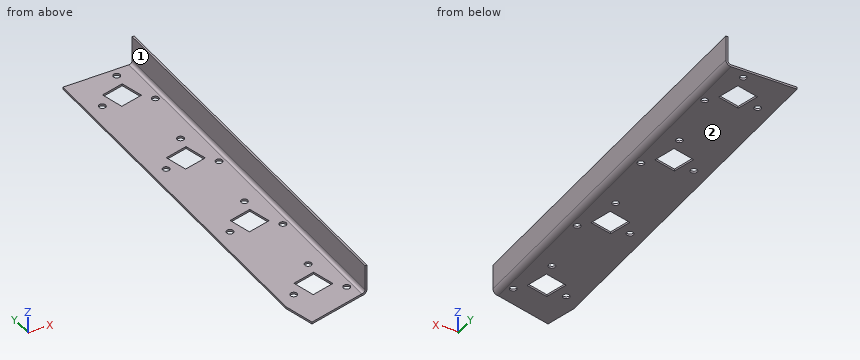
Autodesk Inventor part; units mm, degrees
ref_plane "YZ Plane" through (0, 0, 0) normal (1, 0, 0) x (0, 1, 0)
ref_plane "XZ Plane" through (0, 0, 0) normal (0, 1, 0) x (-1, 0, 0)
ref_plane "XY Plane" through (0, 0, 0) normal (0, 0, 1) x (1, 0, 0)
sketch "Sketch1" plane through (0, 0, 0) normal (0, 0, 1) x (1, 0, 0)
  line L0 (-52.5, 292) -> (52.5, 292)
  line L1 (52.5, 292) -> (52.5, -292)
  line L2 (52.5, -292) -> (-52.5, -292)
  line L3 (-52.5, -292) -> (-52.5, 292)
  line L4 (-52.5, 292) -> (52.5, -292) construction
  point P0 (0, 0)
  point P1 (0, 0)
  dimension "d0" = 105
  dimension "d1" = 584
extrude "Plate1" add sketch "Sketch1" along normal blind 3
sketch "Sketch4" plane through (49.5, 292, 0) normal (1, 0, 0) x (0, 1, 0)
  line L0 (-584, 0) -> (0, 0)
  line L1 (0, 0) -> (0, 45)
  line L2 (0, 45) -> (-584, 45)
  line L3 (-584, 45) -> (-584, 0)
edge flange "Flange1" height 45 angle 90 thickness 3 bend radius 5 thickness toward (1, 0, 0) relief round relief width 3 relief depth 1.5 edges at (52.5, 0, 3) wall of the first edge with corners at (49.5, -292, 0) (49.5, 292, 0) (49.5, 292, 45) (49.5, -292, 45)
bend "Bend1"
corner "Corner1"
sketch "Sketch5" plane through (0, 0, 0) normal (0, 0, -1) x (-1, 0, 0)
  line L0 (-44.5, 292) -> (-44.5, -292)
  line L1 (52.5, -292) -> (-44.5, -292)
  line L2 (52.5, 292) -> (52.5, -292)
  line L3 (-44.5, 292) -> (52.5, 292)
  line L4 (52.5, -292) -> (52.5, -316.1848)
  line L5 (-44.5, -292) -> (52.5, -292)
  line L6 (52.5, -316.1848) -> (-44.5, -292)
  point P0 (0, 0)
  dimension "d25" = 14
extrude "Extrusion2" add sketch "Sketch5" against normal up to surface (3 mm away) contours L1 L4 L6
sketch "Sketch6" plane through (0, 0, 0) normal (0, 0, -1) x (-1, 0, 0)
  line L0 (-44.5, 292) -> (-44.5, -292) construction
  line L1 (-44.5, -292) -> (52.5, -316.1848)
  line L2 (52.5, 292) -> (52.5, -316.1848)
  line L3 (-44.5, 292) -> (52.5, 292) construction
  line L4 (41.1893, -313.3647) -> (52.5, -268)
  line L5 (-44.5, -292) -> (52.5, -316.1848)
  point P0 (0, 0)
  dimension "d45" = 560
extrude "Cut1" cut sketch "Sketch6" against normal blind 3
sketch "Sketch7" plane through (0, 0, 0) normal (0, 0, 1) x (1, 0, 0)
  line L0 (44.5, -292) -> (-41.1893, -313.3647)
  circle A0 centre (36.1472, -268.8326) radius 5.05
  line L1 (36.1472, -268.8326) -> (19.2126, -200.9119) construction
  line L2 (24.6363, -253.6668) -> (16.1691, -219.7064)
  circle A1 centre (19.2126, -200.9119) radius 5.05
  line L3 (-30.5378, -249.3875) -> (36.1472, -268.8326) construction
  line L4 (24.6363, -253.6668) -> (-17.7913, -228.1737) construction
  line L5 (16.1691, -219.7064) -> (-17.7913, -228.1737)
  line L6 (-9.324, -262.1341) -> (24.6363, -253.6668)
  line L7 (16.1691, -219.7064) -> (-9.324, -262.1341) construction
  line L8 (-17.7913, -228.1737) -> (-9.324, -262.1341)
  line L9 (20.4027, -236.6866) -> (-30.5378, -249.3875) construction
  line L10 (19.2126, -200.9119) -> (-30.5378, -249.3875) construction
  circle A2 centre (-30.5378, -249.3875) radius 5.05
  point P0 (0, 0)
  point P1 (3.4225, -240.9203)
  dimension "d32" = 35
  dimension "d33" = 35
  dimension "d34" = 10.1
  dimension "d35" = 70
  dimension "d36" = 60
  dimension "d37" = 25
  dimension "d38" = 10
  dimension "d39" = 42
extrude "Extrusion3" cut sketch "Sketch7" along normal through all
pattern_linear "Rectangular Pattern1" count 4 spacing 160 along (0, 1, 0) of "Extrusion3"
equation "\"d0\" = RIDGE_1_hight"
equation "\"d25\" = RIDGE_1_angle"
equation "\"d45\" = RIDGE_1_lenth"
equation "\"d30\" = Thickness"
equation "\"d33\" = d32"
equation "\"d2\" = Thickness"
equation "\"d15\" = BendReliefWidth"
equation "\"d16\" = BendReliefDepth"
equation "\"d17\" = MinimumRemnant"
equation "\"d18\" = TransitionRadius"
equation "\"d21\" = BendRadius"
equation "\"d22\" = CornerReliefSize"
equation "\"d23\" = GapSize"
equation "\"d24\" = JacobiRadiusSize"
equation "\"BendReliefWidth\" = Thickness"
equation "\"BendReliefDepth\" = 0.5 * Thickness"
equation "\"CornerReliefSize\" = 4 * Thickness"
equation "\"MinimumRemnant\" = 2 * Thickness"
equation "\"TransitionRadius\" = BendRadius"
equation "\"JacobiRadiusSize\" = BendRadius"
equation "\"GapSize\" = Thickness"
properties part number "DS-B-103 Ridge top" material "Stainless Steel"
For this review, take the finished solid that the model builds, in its own axes (mm). Face numbers are marked on the shaded views. A direction names the side the tool comes from. Coordinates: 2 decimals unless noted, no trailing zeros. Write each loop counter-clockwise with the first axis right and the second up, starting at its lowest first coordinate (ties: lowest second). Pieces come first, ordered by that corner, then holes.
(1) Add section B-B on x = 2.5. Give the boundary of the cut face in (y, z).
(2) Add section A-A on y = 193. Give the boundary of the cut face in (x, z), then the cut area to 3 significant figures.
(3) For pin 1 Ø8 at (x, y) = (-30.54, 230.61) entering from -Z; pin 2 Ø2 at (y, z) = (140.5, 5) entering from -X; pin 3 Ø16 at (x, y) = (-30.54, -249.39) entering from +Z; pin 4 Ø1.5 at (y, z) = (-38.5, 23) entering from -X, all flat-tipped, find the tip position at first contact; note any pin that passes through.
(4) Add section C-C on z = 40. Give the boundary of the cut face in (x, y), then the cut area to 3 significant figures.
(5) Wall thickness on probe 1 along X at (y, z) = (-238, 24); probe 2 along Z at (x, y) = (-37, -119); probe 3 along Z at (x, y) = (47.5, 134): over which ranges is each line inside the solid? List them lowest first.
(6) Tool access review of the marked faces 1 and 2: name each direction out of +Z, -Z, +X, -X, +Y, -Y from which nothing blocks a thin tool from reaching the whole face with its end or side.
Answer sheet:
1. outline: (-302.47, 0) - (-259.19, 0) - (-259.19, 3) - (-302.47, 3) - close; (-223.11, 0) - (-99.19, 0) - (-99.19, 3) - (-223.11, 3) - close; (-63.11, 0) - (60.81, 0) - (60.81, 3) - (-63.11, 3) - close; (96.89, 0) - (220.81, 0) - (220.81, 3) - (96.89, 3) - close; (256.89, 0) - (292, 0) - (292, 3) - (256.89, 3) - close
2. outline: (-52.5, 0) - (44.5, 0) arc R8 ccw to (52.5, 8) - (52.5, 45) - (49.5, 45) - (49.5, 8) arc R5 cw to (44.5, 3) - (-52.5, 3) - close
2. area: 433 mm2
3. pin 1: passes through
3. pin 2: stops at x = 47.5
3. pin 3: stops at z = 3
3. pin 4: stops at x = 49.5
4. outline: (49.5, -292) - (52.5, -292) - (52.5, 292) - (49.5, 292) - close
4. area: 1,750 mm2
5. probe 1: x = 49.5 to 52.5
5. probe 2: z = 0 to 3
5. probe 3: z = 0.58 to 4
6. face 1: +Z, -X, +Y, -Y
6. face 2: -Z, +X, -X, +Y, -Y
